Geometry check sheet. Reference: the model listing, model coordinates, mm. A direction names the side the tool comes from. Coordinates: 2 decimals unless noted, no trailing zeros. Write each loop counter-clockwise with the first axis right and the second up, starting at its lowest first coordinate (ties: lowest second). Pieces come first, ordered by that corner, then holes. Notation, with made-up numbers: (18.5, 37) - (53.5, 37) arc R19 cw to (53.5, 61) - close; hole circle Ø8 at (78.25, 38.25). An arc over 180 degrees is marked (long way). Answer as a JSON object with one key per item and string values. Group by question number.
from build123d import *

# Parameters (mm, degrees)
SKETCH003_R     = 1
PAD001_DEPTH    = 5
SKETCH_R        = 4.5
PAD_DEPTH       = 10
SKETCH001_R     = 3.1
POCKET_DEPTH    = 6.5
POCKET001_DEPTH = 3.501


with BuildPart() as hole:
    # Sketch003 → Pad001 (new body, symmetric)
    with BuildSketch(Plane.YZ):
        with Locations((0, 7)):
            Circle(SKETCH003_R)
    extrude(amount=PAD001_DEPTH, both=True)


with BuildPart() as cut:
    # Sketch (on Part) → Pad (new body)
    with BuildSketch(Plane.XY):
        Circle(SKETCH_R)
    extrude(amount=PAD_DEPTH)

    # Sketch001 (on Face3 of Pad) → Pocket (cut)
    with BuildSketch(Plane.XY.offset(10)):
        Circle(SKETCH001_R)
    extrude(amount=-POCKET_DEPTH, mode=Mode.SUBTRACT)

    # Sketch002 (on Face5 of Pocket) → Pocket001 (cut, through all)
    with BuildSketch(Plane.XY.offset(3.5)):
        with BuildLine():
            Line((2.25, 2.132487), (2.25, -2.367513))
            ThreePointArc((-2.25, -2.367513), (0, -3.266132), (2.25, -2.367513))
            Line((-2.25, -2.367513), (-2.25, 2.132487))
            ThreePointArc((2.25, 2.132487), (0, 3.1), (-2.25, 2.132487))
        make_face()
    extrude(amount=-POCKET001_DEPTH, mode=Mode.SUBTRACT)

    # Cut: cut Hole
    add(hole.part, mode=Mode.SUBTRACT)


solid = cut.part
(1) Material ranges on L1, parallel to Y at x = 0, z = 8.75; L2, parallel to Z at x = 3.7, y = 0; L3, parallel to X at y = 2.25, z = 5, recorded low to high. Write a range as [from, to].
(2) Set-up check for faces 4 (the face through (2.6, 0, 3.5)), 5 (the face through (-0.035, -3.266, 1.774)), 6 (the face through (3, 0, 0)): record each of +Z, -Z, +X, -X, +Y, -Y from which the full face is reachable in a straight line by a thin tool's end or side.
(3) Section check A-A (y = 0). Record the cut outline in (x, z), and give its area (4 significant figures).
(4) Section check D-D (z = 2.25). Record the cut outline in (x, y).
(5) Section check C-C (z = 7). Record the cut outline in (x, y).
(6) Section check B-B (x = 0). Record the cut outline in (y, z).
(7) Draft check along Z on faces 1 (the face through (2.25, 0, 2)), 2 (the face through (-4, 0, 6)), 3 (the face through (-3.1, 1.1, 10)). Enter one of: +Z half, -Z half, draft (parallel to the pull), parting line (faces both ways), or undercut.
(8) Gauge pin test, flat ends, axial feed: pin 1 (1.5 mm diameter, centred on x = 2, z = 8, fed in from -Y); pin 2 (5 mm diameter, centred on y = -3, z = 7.5, fed in from +X); pin 3 (2 mm diameter, centred on x = 1, y = -1, fed in from -Z); pin 4 (0.9 mm diameter, centred on x = 2.5, y = 0, fed in from +Z). Record the tip position at first contact, or that the pin passes through.
Conclusion:
{
 "1": {"L1": "y = [-4.5, -3.1], [3.1, 4.5]", "L2": "z = [0, 6], [8, 10]", "L3": "x = [-3.9, -2.13], [2.13, 3.9]"},
 "2": {"face 4": "+Z", "face 5": "-Z", "face 6": "-Z, +X, -X, +Y, -Y"},
 "3": {"outline": "(-4.5, 0) - (-2.25, 0) - (-2.25, 3.5) - (-3.1, 3.5) - (-3.1, 6) - (-4.5, 6) - close; (-4.5, 8) - (-3.1, 8) - (-3.1, 10) - (-4.5, 10) - close; (2.25, 0) - (4.5, 0) - (4.5, 6) - (3.1, 6) - (3.1, 3.5) - (2.25, 3.5) - close; (3.1, 8) - (4.5, 8) - (4.5, 10) - (3.1, 10) - close", "area": "28.35 mm^2"},
 "4": {"outline": "circle Ø9 at (0, 0); hole (-2.25, -2.37) arc R3.27 ccw to (2.25, -2.37) - (2.25, 2.13) arc R3.1 ccw to (-2.25, 2.13) - close"},
 "5": {"outline": "(-4.39, -1) arc R4.5 ccw to (4.39, -1) - (2.93, -1) arc R3.1 cw to (-2.93, -1) - close; (-4.39, 1) - (-2.93, 1) arc R3.1 cw to (2.93, 1) - (4.39, 1) arc R4.5 ccw to start"},
 "6": {"outline": "(-4.5, 0) - (-3.27, 0) - (-3.27, 3.5) - (-3.1, 3.5) - (-3.1, 10) - (-4.5, 10) - close; (3.1, 0) - (4.5, 0) - (4.5, 10) - (3.1, 10) - close"},
 "7": {"face 1": "draft", "face 2": "undercut", "face 3": "+Z half"},
 "8": {"pin 1": "stops at y = -4.32", "pin 2": "stops at x = 4.47", "pin 3": "passes through", "pin 4": "stops at z = 3.5"}
}
